Print and shaded views of the part. All mm, measured from the part's lowest x, y and z. A direction names the side the tool comes from. Coordinates: 2 decimals unless noted, no trailing zeros. Order: outer loops, then holes, each group sorted by start corner. A loop starts at its lowest first (then second) coordinate and runs counter-clockwise, first axis right, second up. Notation, with made-up numbers: M -16,23 L 0,23 A29 ccw 0,61 Z; hole C 51.25,-32.5 d10. An arc over 180 degrees is marked long. Return JSON: item names as keys, results as strings.
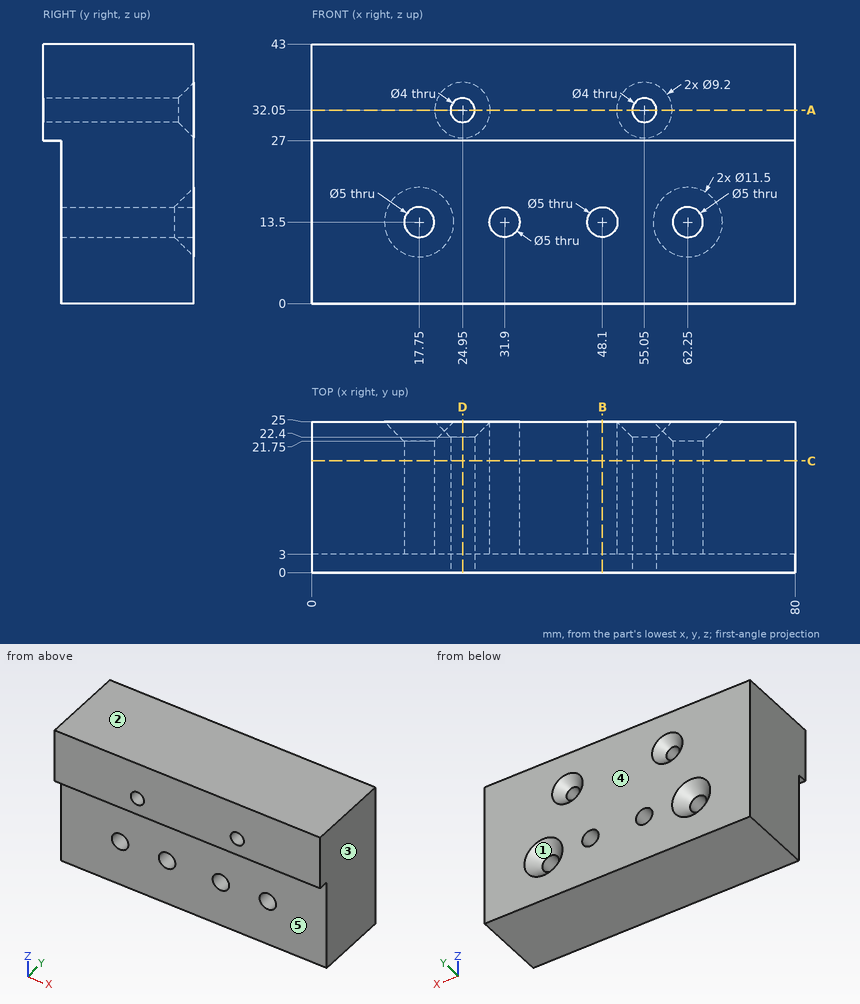
Item 1: Saw through at A-A (z = 32.05). Write the cut outline in (x, y), and give its area (3 significant figures).
Check result:
{"outline": "M 0,0 L 22.95,0 L 22.95,22.4 L 20.35,25 L 0,25 Z; M 26.95,0 L 53.05,0 L 53.05,22.4 L 50.45,25 L 29.55,25 L 26.95,22.4 Z; M 57.05,0 L 80,0 L 80,25 L 59.65,25 L 57.05,22.4 Z", "area": "1,790 mm2"}
Item 2: Wall check: line 1 (X direction, y = 17.5, z = 32.05); line 2 (Z direction, x = 24.95, y = 8); line 3 (Z direction, x = 48.1, y = 8). Give the ranges that are in metal, low to high.
Check result:
{"line 1": "x = 0 to 22.95, 26.95 to 53.05, 57.05 to 80", "line 2": "z = 0 to 30.05, 34.05 to 43", "line 3": "z = 0 to 11, 16 to 43"}
Item 3: 3-axis set-ups, long thin cutter, end or side, ignore diameter. For the marked faces 4 and 5: which of +Z, -Z, +X, -X, +Y, -Y reach the whole face in a straight line?
Check result:
{"face 4": "+Z, -Z, +X, -X, +Y", "face 5": "-Z, +X, -X, -Y"}
Item 4: Saw through at B-B (x = 48.1). Write the cut outline in (y, z).
Check result:
{"outline": "M 0,27 L 3,27 L 3,16 L 25,16 L 25,43 L 0,43 Z; M 3,0 L 25,0 L 25,11 L 3,11 Z"}
Item 5: Pull direction Z, two halves, no side cores. Call the marked faces 1, 2 and 3: +Z half, -Z half, draft (parallel to the pull), parting line (faces both ways), or undercut.
Check result:
{"face 1": "undercut", "face 2": "+Z half", "face 3": "draft"}
Item 6: Saw through at D-D (x = 24.95). Write the cut outline in (y, z), and give its area (3 significant figures).
Check result:
{"outline": "M 0,27 L 3,27 L 3,0 L 25,0 L 25,27.45 L 22.4,30.05 L 0,30.05 Z; M 0,34.05 L 22.4,34.05 L 25,36.65 L 25,43 L 0,43 Z", "area": "887 mm2"}
Item 7: Saw through at C-C (y = 18.5). Write the cut outline in (x, z).
Check result:
{"outline": "M 0,0 L 80,0 L 80,43 L 0,43 Z; hole C 17.75,13.5 d5; hole C 24.95,32.05 d4; hole C 31.9,13.5 d5; hole C 48.1,13.5 d5; hole C 55.05,32.05 d4; hole C 62.25,13.5 d5"}
Item 8: Drop flat-ended pins along their axis: pin 1 Ø4 at (x, y) = (32, 12.5) entering from -Z; pin 2 Ø4 at (x, z) = (31.9, 13.5) entering from +Y; pin 3 Ø6 at (x, z) = (36, 15.5) entering from -Y; pin 4 Ø5 at (x, z) = (24.95, 32.05) entering from +Y. Give the stop position or say it passes through.
Check result:
{"pin 1": "stops at z = 0", "pin 2": "passes through", "pin 3": "stops at y = 3", "pin 4": "stops at y = 22.9"}
